Check sheet for the modelled part. Datum: model origin and axes. Units: mm. A direction names the side the tool comes from. Round coordinates to 2 decimals unless told otherwise and drop trailing zeros. Write each loop counter-clockwise with the first axis right and the second up, starting at its lowest first coordinate (ties: lowest second). Pieces come first, ordered by that corner, then holes. Notation, with made-up numbers: (-18, -24.5) - (33, -24.5) arc R31 cw to (33, 10.5) - close; hole circle Ø6 at (-7.75, 77.5). An arc over 180 degrees is marked (long way). Answer as a JSON object with one key per item and string values. Group by question number.
Item 1: Release check for a two-part mould opening along Y. For faces 1 (the flat face through (3, 17, 1)), 2 (the flat face through (2, -0.75, 6)), 3 (the flat face through (1.479, 49.554, -4.809)) record: pulls with the +Y half, pulls with the -Y half, needs draft (parallel to the pull), parting line crosses it, or undercut.
Item 2: Sectioned sample at C-C on y = 43.5. Record the boundary of the cut face in (x, z), plus the area to 3 significant figures.
Item 3: Thickness scan on line 1 (Y direction, x = 0.6, z = -4.5); line 2 (Y direction, x = 2.5, z = -1.5); line 3 (Y direction, x = 0.8, z = -11). Record the ranges inside material, lowest first.
Item 4: Sectioned sample at B-B on z = 9. Record the boundary of the cut face in (x, y).
Item 5: Set-up check for faces 4 (the cylindrical face through (1.479, 46.226, -7.748)), 5 (the cylindrical face through (1.479, 1.929, 4.613)), 6 (the flat face through (1.479, 51.356, 16.573)), 7 (the flat face through (1.48, 35.45, -6.59)), 8 (the flat face through (0, 17, 1)): record each of +Z, -Z, +X, -X, +Y, -Y from which the full face is reachable in a straight line by a thin tool's end or side.
Item 6: Gauge pin test, flat ends, axial feed: P1, Ø0.7, axis at x = 1, y = 5.5, coming from the -Z side; P2, Ø1.2, axis at x = 1, y = 5.5, coming from the +Z side; P3, Ø5, axis at y = 19, z = -5.5, coming from the -X side; P4, Ø1.2, axis at x = 2, y = 0, coming from the +Z side. Record the tip position at first contact, or that the pin passes through.
Item 7: Sectioned sample at A-A on y = 0. Record the boundary of the cut face in (x, z).
```python
from build123d import *

# Parameters (mm, degrees)
SKETCH1_R           = 5
BOSS_EXTRUDE1_DEPTH = 3
CUT_EXTRUDE1_DEPTH  = 53.748723346
CIRPATTERN1_COUNT   = 8
BOSS_EXTRUDE2_DEPTH = 3
CIRPATTERN2_COUNT   = 6
CIRPATTERN2_ANGLE   = 35.051
FILLET1_R           = 10


with BuildPart() as part:
    # Sketch1 → Boss-Extrude1 (new body)
    with BuildSketch(Plane.YZ):
        with BuildLine():
            ThreePointArc((-15, 0), (-0.831277496, -14.976948211), (14.907863697, -1.66))
            Line((14.907863697, -1.66), (26.907863697, -1.66))
            Line((26.907863697, -1.66), (44.228371772, -11.66))
            ThreePointArc((44.228371772, -11.66), (49.257804904, 2.141068881), (49.25938105, 16.83))
            ThreePointArc((49.25938105, 16.83), (17.396021386, 10.510227399), (-15, 12.9))
            Line((-15, 12.9), (-15, 0))
        make_face()
        with Locations(Location((0, 0, 0), (0, 0, 270))):
            Circle(SKETCH1_R, mode=Mode.SUBTRACT)
    extrude(amount=BOSS_EXTRUDE1_DEPTH)

    # Sketch1_3 → Cut-Extrude1 (cut, symmetric)
    with BuildSketch(Plane.YZ):
        with BuildLine():
            Line((0.75, 6.44), (-0.75, 6.44))
            Line((-0.75, 6.44), (-0.75, 4.943429983))
            ThreePointArc((-0.75, 4.943429983), (0, 5), (0.75, 4.943429983))
            Line((0.75, 4.943429983), (0.75, 6.44))
        make_face()
    cut_extrude1 = extrude(amount=CUT_EXTRUDE1_DEPTH, both=True, mode=Mode.SUBTRACT)

    # CirPattern1: Cut-Extrude1 ×8 about axis
    cirpattern1_axis = Axis((0, 0, 0), (1, 0, 0))
    for i in range(1, CIRPATTERN1_COUNT):
        add(cut_extrude1.rotate(cirpattern1_axis, i * 360 / CIRPATTERN1_COUNT), mode=Mode.SUBTRACT)

    # Sketch1_4 → Boss-Extrude2 (add)
    with BuildSketch(Plane.YZ):
        with BuildLine():
            ThreePointArc((49.25938105, 16.83), (49.541442906, 14.996225218), (49.74274412, 13.151837335))
            Line((49.74274412, 13.151837335), (53.53256333, 15.322287261))
            ThreePointArc((53.53256333, 15.322287261), (53.466194285, 15.822664237), (53.394369482, 16.322287261))
            Line((53.394369482, 16.322287261), (49.25938105, 16.83))
        make_face()
    boss_extrude2 = extrude(amount=BOSS_EXTRUDE2_DEPTH)

    # CirPattern2: Boss-Extrude2 ×6 about axis
    cirpattern2_axis = Axis((0, 7.641692502, 9.49), (-1, 0, 0))
    for i in range(1, CIRPATTERN2_COUNT):
        add(boss_extrude2.rotate(cirpattern2_axis, i * CIRPATTERN2_ANGLE / (CIRPATTERN2_COUNT - 1)))

    # Fillet1
    fillet1_edges = [part.edges().sort_by_distance(p)[0] for p in [
        (1.5, -15, 12.9),
    ]]
    fillet(fillet1_edges, radius=FILLET1_R)


solid = part.part
```
Completed:
{
 "1": {"face 1": "needs draft", "face 2": "undercut", "face 3": "pulls with the +Y half"},
 "2": {"outline": "(0, -11.24) - (3, -11.24) - (3, 15.01) - (0, 15.01) - close", "area": "78.8 mm²"},
 "3": {"line 1": "-14.31 to -4.61, -3.44 to -2.18, 2.18 to 3.44, 4.61 to 14.31, 31.83 to 49.11", "line 2": "-14.92 to -4.77, 4.77 to 52.58", "line 3": "-10.2 to 10.2, 43.09 to 48.81"},
 "4": {"outline": "(0, -11.19) - (3, -11.19) - (3, 52.29) - (0, 52.29) - close"},
 "5": {"face 4": "+X, -X, +Y", "face 5": "+X, -X", "face 6": "+Z, +X, -X, +Y", "face 7": "-Z, +X, -X", "face 8": "+Z, -Z, -X, +Y, -Y"},
 "6": {"P1": "z = -14.09", "P2": "z = 10.39", "P3": "through", "P4": "z = 10.75"},
 "7": {"outline": "(0, -15) - (3, -15) - (3, -6.44) - (0, -6.44) - close; (0, 6.44) - (3, 6.44) - (3, 10.7) - (0, 10.7) - close"}
}
